Autodesk Inventor part; units mm, degrees
ref_plane "YZ Plane" through (0, 0, 0) normal (1, 0, 0) x (0, 1, 0)
ref_plane "XZ Plane" through (0, 0, 0) normal (0, 1, 0) x (-1, 0, 0)
ref_plane "XY Plane" through (0, 0, 0) normal (0, 0, 1) x (1, 0, 0)
sketch "Sketch1" plane through (0, 0, 0) normal (0, 0, 1) x (1, 0, 0)
  circle A0 centre (4.5, -4.5) radius 1.75
  circle A1 centre (14.3, -21.9) radius 1.75
  line L0 (15.3, -26.4) -> (3.5, -26.4)
  line L1 (0, -22.9) -> (0, -3.5)
  line L2 (18.8, -22.9) -> (18.8, -19.7088)
  line L3 (5.0373, 0) -> (3.5, 0)
  arc A2 (3.5, 0) -> (0, -3.5) centre (3.5, -3.5) ccw
  arc A3 (7.956, -1.5683) -> (5.0373, 0) centre (5.0373, -3.5) ccw
  arc A4 (15.3, -26.4) -> (18.8, -22.9) centre (15.3, -22.9) ccw
  arc A5 (0, -22.9) -> (3.5, -26.4) centre (3.5, -22.9) ccw
  line L4 (14.3, -21.9) -> (14.3, -17.4)
  line L5 (18.8, -19.7088) -> (18.8, -18.5234)
  line L6 (18.19, -16.5491) -> (7.956, -1.5683)
  arc A6 (18.8, -18.5234) -> (18.19, -16.5491) centre (15.3, -18.5234) ccw
  point P0 (0, 0)
  point P1 (6.9181, 0)
  point P2 (4.2687, 0)
  dimension "d0" = 3.5
  dimension "d1" = 3.5
  dimension "d34" = 4.5
  dimension "d35" = 4.5
  dimension "d38" = 6.9181
  dimension "d39" = 3.5
  dimension "d46" = 3.5
  dimension "d66" = 9.8
  dimension "d67" = 17.4
  dimension "d68" = 19.97
  dimension "d69" = 4.5
  dimension "d70" = 4.5
  dimension "d71" = 4.5
  dimension "d72" = 3.5
extrude "Extrusion5" add sketch "Sketch1" along normal blind 2
sketch "Sketch5" plane through (0, 0, 2) normal (0, 0, 1) x (1, 0, 0)
  line L0 (0, -3.5) -> (0, -22.9)
  line L1 (0, -14.5491) -> (16.1836, -14.5491)
  line L2 (0, -14.5491) -> (0, -16.5491)
  line L3 (0, -16.5491) -> (17.3511, -16.5491)
  line L4 (0, -14.5491) -> (16.8237, -14.5491)
  line L5 (18.19, -16.5491) -> (7.956, -1.5683)
  line L6 (18.19, -16.5491) -> (0, -16.5491)
  line L7 (0, -3.5) -> (0, -22.9)
  line L8 (18.19, -16.5491) -> (16.8237, -14.5491)
  point P0 (0, 0)
  point P1 (0, -16.5491)
  dimension "d42" = 2
  dimension "d76" = 0
extrude "Extrusion6" add sketch "Sketch5" along normal blind 30
fillet "Fillet2" radius 2 3 edges at (0, -15.5491, 32) (8.4119, -14.5491, 2) (9.095, -16.5491, 2)
sketch "Sketch6" plane through (0, -22.9, 0) normal (-1, 0, 0) x (0, 0, 1)
  line L0 (4, 6.3509) -> (30, 6.3509)
  line L1 (2, 2.75) -> (2, -0.75)
  line L2 (2, 6.3509) -> (2, 1.3509)
  line L3 (2, 6.3509) -> (2, 1.3509)
  line L4 (2, 1.3509) -> (21.3649, 6.3509)
  line L5 (21.3649, 6.3509) -> (2, 6.3509)
  point P0 (0, 22.9)
  point P1 (2, 2.75)
  dimension "d73" = 5
  dimension "d74" = 5
  dimension "d75" = 20
extrude "Extrusion7" add sketch "Sketch6" against normal blind 2
sketch "Sketch7" plane through (0, -14.5491, 4) normal (0, 1, 0) x (1, 0, 0)
  circle A0 centre (8.4575, -5) radius 1.5
  circle A1 centre (8.4575, -23) radius 1.5
  line L0 (0, 0) -> (0, -26)
  line L1 (16.8237, -28) -> (2, -28)
  line L2 (0, 0) -> (16.8237, 0)
  line L3 (16.8237, 0) -> (16.8237, -28)
  point P0 (0, 4)
  point P1 (13.7853, -28)
  dimension "d54" = 3
  dimension "d55" = 3
  dimension "d56" = 18
  dimension "d58" = 8.4575
  dimension "d59" = 8.4575
  dimension "d62" = 5
  dimension "d63" = 5
  dimension "d78" = 16.8237
extrude "Extrusion8" cut sketch "Sketch7" against normal blind 2
fillet "Fillet3" radius 2 1 edges at (17.5069, -15.5491, 32)
properties part number "BLTouch Mount"
For this review, take the finished solid that the model builds, in its own axes (mm). A direction names the side the tool comes from. Round coordinates to 2 decimals unless told otherwise and drop trailing zeros. Loops run counter-clockwise (first coordinate to the right, second up) from the corner with the lowest first, then second, coordinate; pieces in that order, holes last. Notation, with made-up numbers: (59, 80) - (89, 80) arc R26 cw to (89, 119) - close; hole circle Ø7 at (11, 68.25). An arc over 180 degrees is marked (long way). Answer as CSV lines item,"result".
(1) Consider section A-A on x = 4.5. Give the boundary of the cut face in (y, z), then the cut area to 3 significant figures.
Checked values:
outline,"(-26.4, 0) - (-6.25, 0) - (-6.25, 2) - (-12.55, 2) arc R2 cw to (-14.55, 4) - (-14.55, 32) - (-16.55, 32) - (-16.55, 4) arc R2 cw to (-18.55, 2) - (-26.4, 2) - close; (-2.75, 0) - (0, 0) - (0, 2) - (-2.75, 2) - close"
area,"108 mm2"
(2) Mouldability with a two-part tool opening along X and no side actions: class faces 4 (the face through (4, 0, 1)), 5 (the face through (15.11, -20.35, 0.99)), 6 (the face through (2, -18, 9)) as +X half, -X half, draft (parallel to the pull), parting line (faces both ways), or undercut.
Checked values:
face 4,"draft"
face 5,"undercut"
face 6,"+X half"
(3) Consider section D-D on x = 10.5. Give the boundary of the cut face in (y, z).
Checked values:
outline,"(-26.4, 0) - (-5.29, 0) - (-5.29, 2) - (-12.55, 2) arc R2 cw to (-14.55, 4) - (-14.55, 32) - (-16.55, 32) - (-16.55, 4) arc R2 cw to (-18.55, 2) - (-26.4, 2) - close"
(4) Consider section B-B on y = -4.5. Give the boundary of the cut face in (x, z), then the cut area to 3 significant figures.
Checked values:
outline,"(0, 0) - (2.75, 0) - (2.75, 2) - (0, 2) - close; (6.25, 0) - (9.96, 0) - (9.96, 2) - (6.25, 2) - close"
area,"12.9 mm2"
(5) Wall thickness on line 1 (Y direction, x = 4.5, z = 1.15); line 2 (Z direction, x = 12.5, y = -19.25); line 3 (Y direction, x = 2.75, z = 6.5): over which ranges is each line inside the solid? List them lowest first.
Checked values:
line 1,"y = -26.4 to -6.25, -2.75 to 0"
line 2,"z = 0 to 2"
line 3,"y = -16.55 to -14.55"
(6) Consider section C-C on z = 27. Give the boundary of the cut face in (x, y).
Checked values:
outline,"(0, -16.55) - (6.96, -16.55) - (6.96, -14.55) - (0, -14.55) - close; (9.96, -16.55) - (18.19, -16.55) - (16.82, -14.55) - (9.96, -14.55) - close"
(7) Insertion check: P1, Ø5, axis at x = 16.5, y = -7.5, coming from the +Z side; P2, Ø4, axis at y = -20, z = 15, coming from the +X side; P3, Ø9, axis at x = 7, z = 19, coming from the -Y side; P4, Ø5, axis at x = 6, y = -3.5, coming from the +Z side. Each pin has a flat end and moves straight along its axis. Give the tip position at first contact, or say it passes through.
Checked values:
P1,"passes through"
P2,"stops at x = 2"
P3,"stops at y = -16.55"
P4,"stops at z = 2"
(8) Tool access review of faces 1 (the face through (6, -8, 2)), 2 (the face through (9, -22, 2)), 3 (the face through (18.64, -17.48, 1.08)): name each direction out of +Z, -Z, +X, -X, +Y, -Y from which nothing blocks a thin tool from reaching the whole face with its end or side.
Checked values:
face 1,"+Z, +X, -X, +Y"
face 2,"+Z, +X, -Y"
face 3,"+Z, -Z, +X, +Y"
